from build123d import *

# Parameters (mm, degrees)
F5_DEPTH = 20
F3_R     = 3.5
F6_DEPTH = 20
F1_R     = 5.5
F7_DEPTH = 20


with BuildPart() as f5:
    # F4 (on Top) → F5 (new body)
    with BuildSketch(Plane.XY):
        with BuildLine():
            Line((-15.51383, -6.837761), (-2.140489, -9.768229))
            ThreePointArc((-2.140489, -9.768229), (10, 0), (-2.140489, 9.768229))
            Line((-2.140489, 9.768229), (-15.51383, 6.837761))
            ThreePointArc((-15.51383, 6.837761), (-21.015487, 0), (-15.51383, -6.837761))
        make_face()
    extrude(amount=F5_DEPTH)

    # F3 (on Top) → F6 (cut)
    with BuildSketch(Plane.XY):
        with Locations((-14, 0)):
            Circle(F3_R)
    extrude(amount=F6_DEPTH, mode=Mode.SUBTRACT)

    # F1 (on Top) → F7 (cut)
    with BuildSketch(Plane.XY):
        Circle(F1_R)
    extrude(amount=F7_DEPTH, mode=Mode.SUBTRACT)


solid = f5.part
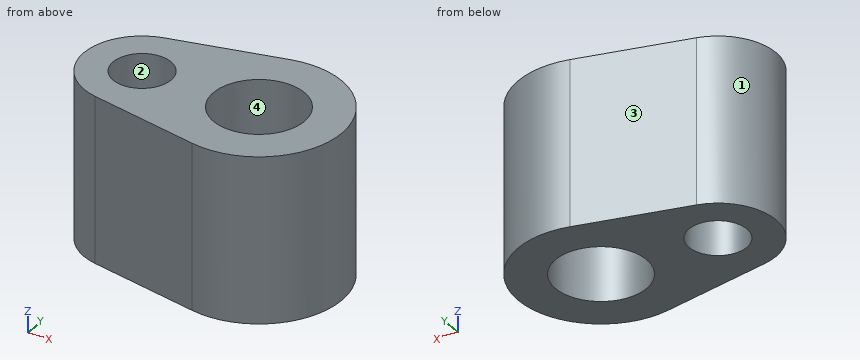
Geometry check sheet. Reference: the model listing, model coordinates, mm. Face numbers are marked on the shaded views. Round coordinates to 2 decimals unless told otherwise and drop trailing zeros. Order: outer loops, then holes, each group sorted by start corner. A loop starts at its lowest first (then second) coordinate and runs counter-clockwise, first axis right, second up. Notation, with made-up numbers: (20, 24) -> (52, 24) arc R38 ccw to (52, 63) -> close; hole circle Ø1 at (61, 4). An arc over 180 degrees is marked (long way). Use one line per item in the form item = value.
1. Mould release check, pull along Y, two halves, no side actions. Record for the marked faces 1, 2, 3 and 4: pulls with the +Y half, pulls with the -Y half, needs draft (parallel to the pull), parting line crosses it, or undercut.
Working result:
face_1 = parting line crosses it
face_2 = undercut
face_3 = pulls with the +Y half
face_4 = undercut
2. Cross-section at B-B, the plane x = 0. Enter the section's corners in (y, z), plus the area to 3 significant figures.
Working result:
outline = (-10, 0) -> (-5.5, 0) -> (-5.5, 20) -> (-10, 20) -> close; (5.5, 0) -> (10, 0) -> (10, 20) -> (5.5, 20) -> close
area = 180 mm^2
3. Scan lines: line 1 along X through (y, z) = (-2.75, 13); line 2 along Y through (x, z) = (0, 6.75); line 3 along X through (y, z) = (4.5, 2.5). Record each from-to range of solid material in increasing order. Write a range as from..to.
Working result:
line_1 = -20.45..-16.17, -11.83..-4.76, 4.76..9.61
line_2 = -10..-5.5, 5.5..10
line_3 = -19.38..-3.16, 3.16..8.93
4. Cross-section at A-A, the plane y = 0. Enter the section's corners in (x, z).
Working result:
outline = (-21.02, 0) -> (-17.5, 0) -> (-17.5, 20) -> (-21.02, 20) -> close; (-10.5, 0) -> (-5.5, 0) -> (-5.5, 20) -> (-10.5, 20) -> close; (5.5, 0) -> (10, 0) -> (10, 20) -> (5.5, 20) -> close
5. Cross-section at D-D, the plane y = -4.5. Enter the section's corners in (x, z).
Working result:
outline = (-19.38, 0) -> (-3.16, 0) -> (-3.16, 20) -> (-19.38, 20) -> close; (3.16, 0) -> (8.93, 0) -> (8.93, 20) -> (3.16, 20) -> close
6. Go/stop test with flat-tipped pins: pin 1 (2 mm diameter, centred on x = -15, z = 18, fed in from -Y); pin 2 (10 mm diameter, centred on x = -9.5, z = 14, fed in from -Y). Record where each tip stops, or that it passes through.
Working result:
pin_1 = -7.17
pin_2 = -9.25
7. Cross-section at C-C, the plane z = 13. Enter the section's corners in (x, y).
Working result:
outline = (-15.51, -6.84) -> (-2.14, -9.77) arc R10 ccw (long way) to (-2.14, 9.77) -> (-15.51, 6.84) arc R7 ccw to start; hole circle Ø7 at (-14, 0); hole circle Ø11 at (0, 0)
